```python
from build123d import *

# Parameters (mm, degrees)
F0_W      = 100
F0_H      = 100
F1_DEPTH  = 100
F3_DEPTH  = 100
F5_COUNT  = 2
F5_ANGLE  = 90
F6_T      = -1
F7_W      = 1.4
F7_H      = 100
F8_DEPTH  = 100
F10_DEPTH = 2
F11_COUNT = 4


with BuildPart() as f1:
    # F0 (on Top) → F1 (new body)
    with BuildSketch(Plane.XY):
        Rectangle(F0_W, F0_H)
    extrude(amount=F1_DEPTH)

    # F2 (on face) → F3 (join)
    with BuildSketch(Plane.XZ.offset(50)):
        Polygon((-50, 0), (-50, 100), (-147.9795897113, 100), align=None)
        Polygon((147.9795897113, 100), (50, 100), (50, 0), align=None)
    extrude(amount=-F3_DEPTH)

    # F5: F1 ×2 about axis
    f5_axis = Axis((0, 0, 92.5767719746), (0, 0, 1))


with BuildPart() as f1_1:
    add(f1.part)
    for i in range(1, F5_COUNT):
        add(f1.part.rotate(f5_axis, i * F5_ANGLE / (F5_COUNT - 1)))

    # F6
    f6_openings = [f1_1.faces().sort_by_distance(p)[0] for p in [
        (0, 0, 100),
    ]]
    offset(amount=F6_T, openings=f6_openings, kind=Kind.INTERSECTION)

    # F7 (on face) → F8 (join)
    with BuildSketch(Plane.XY.offset(100)):
        with Locations((-147.2795897113, 0)):
            Rectangle(F7_W, F7_H)
    extrude(amount=F8_DEPTH)

    # F9 (on face) → F10 (cut)
    with BuildSketch(Plane(origin=(-147.9795897113, 0, 0), x_dir=(0, -1, 0), z_dir=(-1, 0, 0))):
        Polygon((-50, 200), (-50, 100), (0, 150), (50, 100), (50, 200), align=None)
    extrude(amount=-F10_DEPTH, mode=Mode.SUBTRACT)

    # F11: F1 ×4 about axis
    f11_axis = Axis((0, 0, 92.5767719746), (0, 0, 1))


with BuildPart() as f1_2:
    add(f1_1.part)
    for i in range(1, F11_COUNT):
        add(f1_1.part.rotate(f11_axis, i * 360 / F11_COUNT))


solid = f1_2.part
```
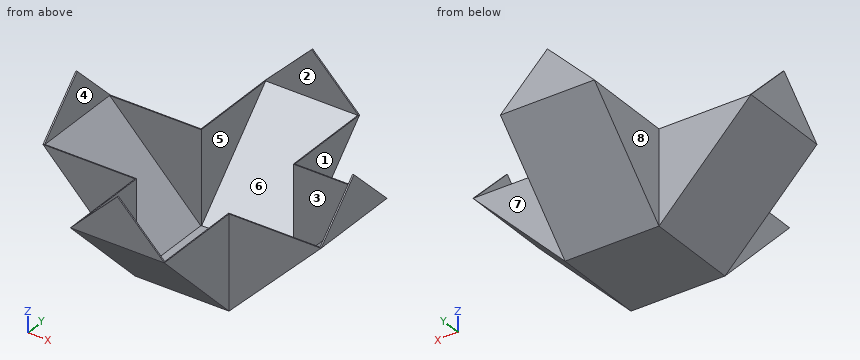
CAD build for the part. Positions are in the model's coordinates, mm. Face numbers are marked on the shaded views. A direction names the side the tool comes from. Round coordinates to 2 decimals unless told otherwise and drop trailing zeros. Loops run counter-clockwise (first coordinate to the right, second up) from the corner with the lowest first, then second, coordinate; pieces in that order, holes last. Notation, with made-up numbers: (24, -39.5) - (43, -39.5) arc R29 ccw to (43, -3.5) - close; hole circle Ø1 at (-1.75, 72). An arc over 180 degrees is marked (long way). Return JSON: item names as keys, results as strings. Group by question number.
Q1. Drill centre lines: line 1 along Y through (x, z) = (-28, 117.5); line 2 along Y through (x, z) = (84.5, 57.5). Where is each one in solid material? Low to high. Write a range as [from, to].
Q2. Tool access for the marked faces 1, 2, 3 and 4: list every direction of +Z, -Z, +X, -X, +Y, -Y with a clear straight run to the whole face (end or side of a thin tool).
Q3. Flat gauge pins, fed straight in: pin 1 Ø5 at (x, z) = (-87.5, 47.5) entering from +Y; pin 2 Ø6 at (x, y) = (-35.5, -63) entering from -Z; pin 3 Ø5 at (x, z) = (20.5, 60) entering from +Y. Where does each tip first touch, or does it go through?
Q4. Band-saw the part on B-B on x = -40.5. Give the cut face in (y, z).
Q5. Band-saw the part on C-C on z = 55. Give the cut face in (x, y).
Q6. Band-saw the part on A-A on y = -7. Give the cut face in (x, z), plus the area to 3 significant figures.
Q7. Two-plate mould, pull along Y, no slides. Class the marked faces 5, 6, 7 and 8: +Y half, -Y half, draft (parallel to the pull), parting line (faces both ways), or undercut.
Q8. Band-saw the part on D-D on y = -59.5. Give the cut face in (x, z).
Solutions:
{
 "1": {"line 1": "y = [-147.98, -146.58], [146.58, 147.98]", "line 2": "y = [-50, -49], [49, 50]"},
 "2": {"face 1": "+Z, -Z, +X, +Y", "face 2": "+Z, +X, -X", "face 3": "+Z", "face 4": "+Z, +Y, -Y"},
 "3": {"pin 1": "stops at y = 50", "pin 2": "stops at z = 10.21", "pin 3": "stops at y = 111.24"},
 "4": {"outline": "(-147.98, 100) - (-50, 0) - (50, 0) - (147.98, 100) - (147.98, 109.5) - (146.58, 109.5) - (146.58, 100) - (49.58, 1) - (-49.58, 1) - (-146.58, 100) - (-146.58, 109.5) - (-147.98, 109.5) - close"},
 "5": {"outline": "(-103.89, -50) - (-50, -50) - (-50, -103.89) - (50, -103.89) - (50, -50) - (103.89, -50) - (103.89, 50) - (50, 50) - (50, 103.89) - (-50, 103.89) - (-50, 50) - (-103.89, 50) - close; hole (-102.49, -49) - (-49, -49) - (-49, -102.49) - (49, -102.49) - (49, -49) - (102.49, -49) - (102.49, 49) - (49, 49) - (49, 102.49) - (-49, 102.49) - (-49, 49) - (-102.49, 49) - close"},
 "6": {"outline": "(-147.98, 100) - (-50, 0) - (50, 0) - (147.98, 100) - (147.98, 143) - (146.58, 143) - (146.58, 100) - (49.58, 1) - (-49.58, 1) - (-146.58, 100) - (-146.58, 143) - (-147.98, 143) - close", "area": "499 mm^2"},
 "7": {"face 5": "undercut", "face 6": "undercut", "face 7": "+Y half", "face 8": "draft"},
 "8": {"outline": "(-50, 9.7) - (50, 9.7) - (50, 100) - (49, 100) - (49, 11.12) - (-49, 11.12) - (-49, 100) - (-50, 100) - close"}
}
